Input: part model. Units: mm. Frame: model coordinates. A direction names the side the tool comes from. Round coordinates to 2 decimals unless told otherwise and drop trailing zeros. Order: outer loops, then holes, each group sorted by start corner. A loop starts at its lowest first (then second) coordinate and runs counter-clockwise, first axis right, second up.
Item 1: Cut plane B-B on y = 72. Output: boundary loops of the cut face in (x, z), then the cut area to 3 significant figures.
Item 2: Reachability of faces 1 (the flat face through (0, 64, 3)), 2 (the flat face through (99.8, 29.6, 2)) from +Z, -Z, +X, -X, +Y, -Y: full face, straight path, thin tool, end or side. Return the list, or none.
Item 3: Mould query, pull axis Y, two halves, no side actions, for faces 3 (the flat face through (200, 64, 3)), 4 (the flat face through (99, 130, 3)), 5 (the cylindrical face through (138.153, 77.015, 4.281)). Classes: released by +Y, released by -Y, zero draft, split by the parting line, or undercut.
Item 4: Cut plane C-C on z = 4. Give the number of separate pieces and of enclosed holes in the cut face, then the cut area to 3 significant figures.
Item 5: Cut plane A-A on x = 70.5. Output: boundary loops of the cut face in (y, z).
Item 6: First-contact query: pin 1 (3.5 mm diameter, centred on x = 64.63, y = 29.64, fed in from -Z); pin 2 (1.9 mm diameter, centred on x = 185, y = 80, fed in from +Z). Flat tips, straight axial feed; report the tip coordinate or a pass-through.
Item 7: Line query: L1, parallel to Y at x = 15, z = 2.5; L2, parallel to X at y = 110, z = 4; L3, parallel to Y at x = 25, z = 5. Output: solid intervals per line, ascending.
```python
from build123d import *

# Parameters (mm, degrees)
SKETCH_W     = 200
SKETCH_H     = 130
SKETCH_R     = 35
SKETCH_R_2   = 1.5625
PAD_DEPTH    = 6.5
SKETCH001_R  = 40
POCKET_DEPTH = 4.5
FILLET_R     = 3


with BuildPart() as part:
    # Sketch → Pad (new body)
    with BuildSketch(Plane.XY):
        with Locations((100, 65)):
            Rectangle(SKETCH_W, SKETCH_H)
        with Locations((100, 65)):
            Circle(SKETCH_R, mode=Mode.SUBTRACT)
        with Locations((45, 115)):
            Circle(SKETCH_R_2, mode=Mode.SUBTRACT)
        with Locations((45, 15)):
            Circle(SKETCH_R_2, mode=Mode.SUBTRACT)
        with Locations((155, 115)):
            Circle(SKETCH_R_2, mode=Mode.SUBTRACT)
        with Locations((155, 15)):
            Circle(SKETCH_R_2, mode=Mode.SUBTRACT)
        with Locations((185, 30)):
            Circle(SKETCH_R_2, mode=Mode.SUBTRACT)
        with Locations((135.353085, 100.338453)):
            Circle(SKETCH_R_2, mode=Mode.SUBTRACT)
        with Locations((64.627773, 29.642413)):
            Circle(SKETCH_R_2, mode=Mode.SUBTRACT)
        with Locations((64.64463, 100.35537)):
            Circle(SKETCH_R_2, mode=Mode.SUBTRACT)
        with Locations((135.352442, 29.63292)):
            Circle(SKETCH_R_2, mode=Mode.SUBTRACT)
        with Locations((175, 20)):
            Circle(SKETCH_R_2, mode=Mode.SUBTRACT)
        with Locations((175, 40)):
            Circle(SKETCH_R_2, mode=Mode.SUBTRACT)
        with Locations((185, 50)):
            Circle(SKETCH_R_2, mode=Mode.SUBTRACT)
        with Locations((175, 90)):
            Circle(SKETCH_R_2, mode=Mode.SUBTRACT)
        with Locations((175, 110)):
            Circle(SKETCH_R_2, mode=Mode.SUBTRACT)
        with Locations((185, 80)):
            Circle(SKETCH_R_2, mode=Mode.SUBTRACT)
        with Locations((185, 100)):
            Circle(SKETCH_R_2, mode=Mode.SUBTRACT)
        with Locations((15, 30)):
            Circle(SKETCH_R_2, mode=Mode.SUBTRACT)
        with Locations((25, 20)):
            Circle(SKETCH_R_2, mode=Mode.SUBTRACT)
        with Locations((25, 40)):
            Circle(SKETCH_R_2, mode=Mode.SUBTRACT)
        with Locations((15, 50)):
            Circle(SKETCH_R_2, mode=Mode.SUBTRACT)
        with Locations((25, 90)):
            Circle(SKETCH_R_2, mode=Mode.SUBTRACT)
        with Locations((25, 110)):
            Circle(SKETCH_R_2, mode=Mode.SUBTRACT)
        with Locations((15, 80)):
            Circle(SKETCH_R_2, mode=Mode.SUBTRACT)
        with Locations((15, 100)):
            Circle(SKETCH_R_2, mode=Mode.SUBTRACT)
    extrude(amount=PAD_DEPTH)

    # Sketch001 (on Face31 of Pad) → Pocket (cut)
    with BuildSketch(Plane.XY.offset(6.5)):
        with Locations((100, 65)):
            Circle(SKETCH001_R)
    extrude(amount=-POCKET_DEPTH, mode=Mode.SUBTRACT)

    # Fillet
    fillet_edges = [part.edges().sort_by_distance(p)[0] for p in [
        (200, 0, 3.25),
        (200, 130, 3.25),
        (0, 0, 3.25),
        (0, 130, 3.25),
    ]]
    fillet(fillet_edges, radius=FILLET_R)


solid = part.part
```
From the geometry:
1. outline: (0, 0) - (65.71, 0) - (65.71, 2) - (60.62, 2) - (60.62, 6.5) - (0, 6.5) - close; (134.29, 0) - (200, 0) - (200, 6.5) - (139.38, 6.5) - (139.38, 2) - (134.29, 2) - close
1. area: 808 mm2
2. face 1: +Z, -Z, -X, +Y, -Y
2. face 2: +Z
3. face 3: zero draft
3. face 4: released by +Y
3. face 5: undercut
4. separate pieces: 1
4. enclosed holes: 25
4. area: 20,800 mm2
5. outline: (0, 0) - (46.17, 0) - (46.17, 2) - (37.99, 2) - (37.99, 6.5) - (0, 6.5) - close; (83.83, 0) - (130, 0) - (130, 6.5) - (92.01, 6.5) - (92.01, 2) - (83.83, 2) - close
6. pin 1: stops at z = 0
6. pin 2: passes through
7. L1: y = 0 to 28.44, 31.56 to 48.44, 51.56 to 78.44, 81.56 to 98.44, 101.56 to 130
7. L2: x = 0 to 23.44, 26.56 to 173.44, 176.56 to 200
7. L3: y = 0 to 18.44, 21.56 to 38.44, 41.56 to 88.44, 91.56 to 108.44, 111.56 to 130
